Can you work these out from the model? Positions are in its coordinate system, mm. A direction names the side the tool comes from. Give positions to 0.01 mm unless a question says otherwise; leave off trailing zeros. Loops run counter-clockwise (first coordinate to the right, second up) from the corner with the lowest first, then second, coordinate; pieces in that order, holes last. Notation, with made-up numbers: (46, 3) -> (52, 3) arc R20 ccw to (52, 22) -> close; hole circle Ø2 at (29.5, -19). An arc over 180 degrees is marked (long way). One line per question, with ' | ' between items.
from build123d import *

# Parameters (mm, degrees)
F0_W          = 3
F0_H          = 3
F0_W_2        = 19
F0_H_2        = 20
F0_W_3        = 25
F0_W_4        = 9
F0_H_3        = 10
F1_DEPTH      = 15
F1_DEPTH_BACK = 15


with BuildPart() as f1:
    # F0 (on Front) → F1 (new body, two sides)
    with BuildSketch(Plane.XZ) as f1_sk:
        with Locations((1.5, 1.5)):
            Rectangle(F0_W, F0_H)
        with Locations((12.5, 1.5)):
            Rectangle(F0_W_2, F0_H)
        with Locations((1.5, 13)):
            Rectangle(F0_W, F0_H_2)
        with Locations((23.5, 1.5)):
            Rectangle(F0_W, F0_H)
        with Locations((23.5, 13)):
            Rectangle(F0_W, F0_H_2)
        with Locations((37.5, 1.5)):
            Rectangle(F0_W_3, F0_H)
        Polygon((50, 3), (50, 0), (50, -5), (53, -5), (53, 3), align=None)
        with Locations((51.5, -6.5)):
            Rectangle(F0_W, F0_H)
        with Locations((57.5, -6.5)):
            Rectangle(F0_W_4, F0_H)
        with Locations((63.5, -6.5)):
            Rectangle(F0_W, F0_H)
        with Locations((63.5, -13)):
            Rectangle(F0_W, F0_H_3)
        Polygon((65, -18), (62, -18), (42, -18), (42, -21), (65, -21), align=None)
    extrude(amount=F1_DEPTH)
    extrude(f1_sk.sketch, amount=-F1_DEPTH_BACK)


solid = f1.part
Q1. If we section it at D-D (z = -6.5): Write out the boundary of the cut face in (x, y), plus the area to 3 significant figures.
Entries:
outline: (50, -15) -> (65, -15) -> (65, 15) -> (50, 15) -> close | area: 450 mm²
Q2. If we section it at B-B (z = 5.5): Write out the boundary of the cut face in (x, y), plus the area to 3 significant figures.
Entries:
outline: (0, -15) -> (3, -15) -> (3, 15) -> (0, 15) -> close; (22, -15) -> (25, -15) -> (25, 15) -> (22, 15) -> close | area: 180 mm²
Q3. On a 3-axis mill with a long thin cutter (end or side, diameter ignored), from which of +Z, -Z, +X, -X, +Y, -Y can I reach the whole of each face in a straight line? I mean faces 1 (the face through (56, 0, -8)), 2 (the face through (53, 0, -1)), 3 (the face through (65, 0, -13)), 4 (the face through (42, 0, -19)), 5 (the face through (3, 0, 13)). Say none if no direction works.
Entries:
face 1: -X, +Y, -Y | face 2: +Z, +X, +Y, -Y | face 3: +Z, -Z, +X, +Y, -Y | face 4: -Z, -X, +Y, -Y | face 5: +Z, +Y, -Y
Q4. If we section it at A-A (y = -7.25): Write out the boundary of the cut face in (x, z).
Entries:
outline: (0, 0) -> (50, 0) -> (50, -8) -> (62, -8) -> (62, -18) -> (42, -18) -> (42, -21) -> (65, -21) -> (65, -5) -> (53, -5) -> (53, 3) -> (25, 3) -> (25, 23) -> (22, 23) -> (22, 3) -> (3, 3) -> (3, 23) -> (0, 23) -> close
Q5. For pin 1 Ø10 at (y, z) = (5, 1.5) entering from -X; pin 2 Ø1 at (y, z) = (5, 18) entering from +X; pin 3 Ø8 at (y, z) = (1.5, -11) entering from -X; pin 4 Ø13 at (x, y) = (57.5, -6.5) entering from +Z, each with a flat end and sliding along its axis, tell me the tip position at first contact or that it passes through.
Entries:
pin 1: x = 0 | pin 2: x = 25 | pin 3: x = 50 | pin 4: z = 3
Q6. If we section it at C-C (x = 37): Write out the boundary of the cut face in (y, z).
Entries:
outline: (-15, 0) -> (15, 0) -> (15, 3) -> (-15, 3) -> close
Q7. If we mould it in two halves opening along Z, with no side actions, what happens to faces 6 (the face through (22, 0, 13)), 7 (the face through (62, 0, -13)), 8 (the face through (1, 0, 23)), 9 (the face through (50, 0, -4))? For each: pulls with the +Z half, pulls with the -Z half, needs draft (parallel to the pull), parting line crosses it, or undercut.
Entries:
face 6: needs draft | face 7: undercut | face 8: pulls with the +Z half | face 9: undercut
Q8. If I drill on probe 1 along X at (y, z) = (-3, 6.5); probe 2 along Z at (x, y) = (52.5, -3.5); probe 3 along Z at (x, y) = (47.5, -5), over which ranges is the centre line in solid material (lowest first)? Write a range as from..to.
Entries:
probe 1: 0..3, 22..25 | probe 2: -21..-18, -8..3 | probe 3: -21..-18, 0..3
